The model under review builds one solid part; all positions refer to its coordinate system, in mm. Give positions to 0.01 mm unless a question says otherwise; leave off trailing zeros. Order: outer loops, then holes, each group sorted by start corner. A loop starts at its lowest first (then second) coordinate and runs counter-clockwise, first axis right, second up. Notation, with made-up numbers: (-27, -2) -> (-14, -2) arc R27 cw to (-14, 18) -> close; hole circle Ø10 at (-38.75, -6.5). An arc over 180 degrees is marked (long way). Answer as a JSON object with one key per item and string values. Group by question number.
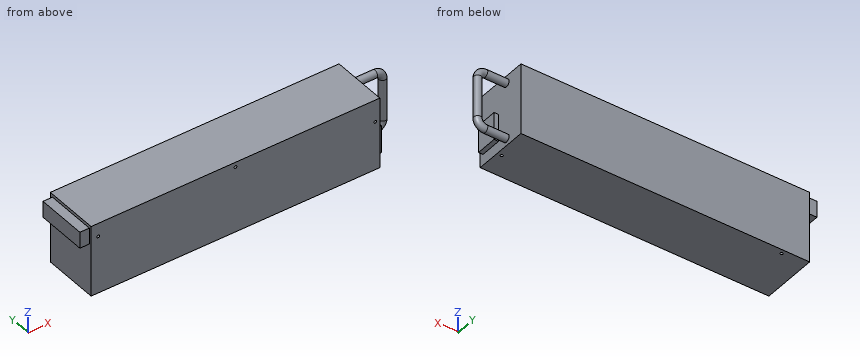
from build123d import *

# Parameters (mm, degrees)
SKETCH1_W           = 325
SKETCH1_H           = 80
BOSS_EXTRUDE1_DEPTH = 63
SKETCH2_R           = 4.2
BOSS_EXTRUDE2_DEPTH = 24
SKETCH3_R           = 4.2
REVOLVE1_ANGLE      = 90
SKETCH4_R           = 4.2
REVOLVE2_ANGLE      = 90
SKETCH5_R           = 4.2
BOSS_EXTRUDE3_DEPTH = 46.7
SKETCH6_W           = 31
SKETCH6_H           = 24
BOSS_EXTRUDE4_DEPTH = 5
SKETCH7_W           = 18.321036957
SKETCH7_H           = 57
BOSS_EXTRUDE5_DEPTH = 10.6
SKETCH8_R           = 1.5
CUT_EXTRUDE1_DEPTH  = 12
SKETCH9_R           = 1.5
CUT_EXTRUDE3_DEPTH  = 12


with BuildPart() as part:
    # Sketch1 → Boss-Extrude1 (new body)
    with BuildSketch(Plane(origin=(0, 0, 0), x_dir=(1, 0, 0), z_dir=(0, 1, 0))):
        with Locations((-162.5, -40)):
            Rectangle(SKETCH1_W, SKETCH1_H)
    extrude(amount=BOSS_EXTRUDE1_DEPTH)

    # Sketch2 → Boss-Extrude2 (add)
    with BuildSketch(Plane(origin=(0, 0, 0), x_dir=(0, 0, -1), z_dir=(1, 0, 0))):
        with Locations((-71.75, 40.5)):
            Circle(SKETCH2_R)
        with Locations((-8.25, 40.5)):
            Circle(SKETCH2_R)
    extrude(amount=BOSS_EXTRUDE2_DEPTH)

    # Sketch3 → Revolve1 (revolve)
    with BuildSketch(Plane(origin=(24, 0, 0), x_dir=(0, 0, -1), z_dir=(1, 0, 0))):
        with Locations((-71.75, 40.5)):
            Circle(SKETCH3_R)
    revolve(axis=Axis((24, 40.5, 63.35), (0, 1, 0)), revolution_arc=REVOLVE1_ANGLE)

    # Sketch4 → Revolve2 (revolve)
    with BuildSketch(Plane(origin=(24, 0, 0), x_dir=(0, 0, -1), z_dir=(1, 0, 0))):
        with Locations((-8.25, 40.5)):
            Circle(SKETCH4_R)
    revolve(axis=Axis((24, 40.5, 16.65), (0, -1, 0)), revolution_arc=REVOLVE2_ANGLE)

    # Sketch5 → Boss-Extrude3 (add)
    with BuildSketch(Plane.XY.offset(16.65)):
        with Locations((32.4, 40.5)):
            Circle(SKETCH5_R)
    extrude(amount=BOSS_EXTRUDE3_DEPTH)

    # Sketch6 → Boss-Extrude4 (add)
    with BuildSketch(Plane(origin=(0, 0, 0), x_dir=(0, 0, -1), z_dir=(1, 0, 0))):
        with Locations((-28, 16.3)):
            Rectangle(SKETCH6_W, SKETCH6_H)
    extrude(amount=BOSS_EXTRUDE4_DEPTH)

    # Sketch7 → Boss-Extrude5 (add)
    with BuildSketch(Plane.ZY.offset(325)):
        with Locations((67.339481522, 31.3)):
            Rectangle(SKETCH7_W, SKETCH7_H)
    extrude(amount=BOSS_EXTRUDE5_DEPTH)

    # Sketch8 → Cut-Extrude1 (cut)
    with BuildSketch(Plane.XZ):
        with Locations((-317, 65)):
            Circle(SKETCH8_R)
        with Locations((-162.5, 74.5)):
            Circle(SKETCH8_R)
        with Locations((-5.25, 55)):
            Circle(SKETCH8_R)
    extrude(amount=-CUT_EXTRUDE1_DEPTH, mode=Mode.SUBTRACT)

    # Sketch9 → Cut-Extrude3 (cut)
    with BuildSketch(Plane(origin=(0, 0, 0), x_dir=(-1, 0, 0), z_dir=(0, 0, -1))):
        with Locations((5.25, 26)):
            Circle(SKETCH9_R)
        with Locations((297, 58)):
            Circle(SKETCH9_R)
    extrude(amount=-CUT_EXTRUDE3_DEPTH, mode=Mode.SUBTRACT)


solid = part.part
1. Take a section at D-D on z = 8.25. State how many separate pieces and enclosed holes the cut face has, plus the area to 3 significant figures.
2. For pin 1 (0.9 mm diameter, centred on x = -163, z = 75, fed in from -Y); pin 2 (12 mm diameter, centred on y = 26, z = 65.5, fed in from +X); pin 3 (1.5 mm diameter, centred on x = -5.5, y = 25.5, fed in from -Z), all flat-tipped, find the tip position at first contact; note any pin that passes through.
3. Take a section at C-C on y = 16. Give the boundary of the cut face in (x, z).
4. Take a section at B-B on z = 29. Give the boundary of the cut face in (x, y), plus the area to 3 significant figures.
5. Take a section at A-A on y = 40.5. Give the boundary of the cut face in (x, z).
6. For probe 1 along Z at (x, y) = (-317, 6); probe 2 along Y at (x, z) = (-297, 4.5); probe 3 along X at (y, z) = (33.5, 22), list the stretches that pass through material, from the lowest coordinate up. Write a range as [from, to].
Checks:
{
 "1": {"separate pieces": "1", "enclosed holes": "2", "area": "20,700 mm2"},
 "2": {"pin 1": "stops at y = 12", "pin 2": "stops at x = 0", "pin 3": "stops at z = 12"},
 "3": {"outline": "(-335.6, 58.18) -> (-325, 58.18) -> (-325, 0) -> (0, 0) -> (0, 12.5) -> (5, 12.5) -> (5, 43.5) -> (0, 43.5) -> (0, 80) -> (-325, 80) -> (-325, 76.5) -> (-335.6, 76.5) -> close"},
 "4": {"outline": "(-325, 0) -> (0, 0) -> (0, 4.3) -> (5, 4.3) -> (5, 28.3) -> (0, 28.3) -> (0, 63) -> (-325, 63) -> close; circle Ø8.4 at (32.4, 40.5)", "area": "20,700 mm2"},
 "5": {"outline": "(-335.6, 58.18) -> (-325, 58.18) -> (-325, 0) -> (0, 0) -> (0, 4.05) -> (24, 4.05) arc R12.6 ccw to (36.6, 16.65) -> (36.6, 63.35) arc R12.6 ccw to (24, 75.95) -> (0, 75.95) -> (0, 80) -> (-325, 80) -> (-325, 76.5) -> (-335.6, 76.5) -> close; hole (0, 12.45) -> (24, 12.45) arc R4.2 ccw to (28.2, 16.65) -> (28.2, 63.35) arc R4.2 ccw to (24, 67.55) -> (0, 67.55) -> close"},
 "6": {"probe 1": "z = [0, 63.5], [66.5, 80]", "probe 2": "y = [0, 56.5], [59.5, 63]", "probe 3": "x = [-325, 0]"}
}
